from build123d import *

# Parameters (mm, degrees)
SKETCH1_W           = 5
SKETCH1_H           = 38.6
BOSS_EXTRUDE1_DEPTH = 3
SKETCH3_W           = 5
SKETCH3_H           = 15
BOSS_EXTRUDE2_DEPTH = 3
SKETCH4_R           = 1.5
CUT_EXTRUDE1_DEPTH  = 4
SKETCH7_W           = 5
SKETCH7_H           = 15
BOSS_EXTRUDE3_DEPTH = 3
SKETCH8_W           = 5
SKETCH8_H           = 2
BOSS_EXTRUDE4_DEPTH = 12
SKETCH10_W          = 5
SKETCH10_H          = 5
BOSS_EXTRUDE5_DEPTH = 3.65


with BuildPart() as part:
    # Sketch1 → Boss-Extrude1 (new body)
    with BuildSketch(Plane.XY):
        Rectangle(SKETCH1_W, SKETCH1_H)
    extrude(amount=BOSS_EXTRUDE1_DEPTH)

    # Sketch3 → Boss-Extrude2 (add)
    with BuildSketch(Plane.XZ.offset(19.3)):
        with Locations((0, 7.5)):
            Rectangle(SKETCH3_W, SKETCH3_H)
    extrude(amount=BOSS_EXTRUDE2_DEPTH)

    # Sketch4 → Cut-Extrude1 (cut)
    with BuildSketch(Plane(origin=(0, -19.3, 0), x_dir=(1, 0, 0), z_dir=(0, 1, 0))):
        with Locations(Location((0, -9.153210304, 0), (0, 0, 270))):
            Circle(SKETCH4_R)
    extrude(amount=-CUT_EXTRUDE1_DEPTH, mode=Mode.SUBTRACT)

    # Sketch7 → Boss-Extrude3 (add)
    with BuildSketch(Plane(origin=(0, 19.3, 0), x_dir=(1, 0, 0), z_dir=(0, 1, 0))):
        with Locations((0, 4.5)):
            Rectangle(SKETCH7_W, SKETCH7_H)
    extrude(amount=BOSS_EXTRUDE3_DEPTH)

    # Sketch8 → Boss-Extrude4 (add)
    with BuildSketch(Plane(origin=(0, 0, 0), x_dir=(-1, 0, 0), z_dir=(0, 0, -1))):
        with Locations((0, 8.6)):
            Rectangle(SKETCH8_W, SKETCH8_H)
    extrude(amount=BOSS_EXTRUDE4_DEPTH)

    # Sketch10 → Boss-Extrude5 (add)
    with BuildSketch(Plane(origin=(0, 0, 0), x_dir=(-1, 0, 0), z_dir=(0, 0, -1))):
        with Locations((0, -4.864250557)):
            Rectangle(SKETCH10_W, SKETCH10_H)
        with Locations((0, -19.864250557)):
            Rectangle(SKETCH10_W, SKETCH10_H)
    extrude(amount=BOSS_EXTRUDE5_DEPTH)


solid = part.part
Geometry check sheet. Reference: the model listing, model coordinates, mm. A direction names the side the tool comes from. Coordinates: 2 decimals unless noted, no trailing zeros. Order: outer loops, then holes, each group sorted by start corner. A loop starts at its lowest first (then second) coordinate and runs counter-clockwise, first axis right, second up. Notation, with made-up numbers: (-6.75, -22) - (43.25, -22) arc R13 cw to (43.25, 1) - close; hole circle Ø6 at (-29, 3). An arc over 180 degrees is marked (long way). One line per item, written item: value.
(1) Depth check by flat-ended pin: pin 1 Ø2.5 at (x, z) = (0, 9.15) entering from +Y; pin 2 Ø1.5 at (x, y) = (-1, -8) entering from +Z; pin 3 Ø6 at (y, z) = (-4, -4) entering from -X; pin 4 Ø1.5 at (x, y) = (-1, -6) entering from -Z. Enter the tip coordinate at first touch or a pass-through.
Data:
pin 1: passes through
pin 2: stops at z = 3
pin 3: stops at x = -2.5
pin 4: stops at z = -3.65
(2) Sectioned sample at C-C (y = 9). Enter the section's corners in (x, z), and give its area (3 significant figures).
Data:
outline: (-2.5, -12) - (2.5, -12) - (2.5, 3) - (-2.5, 3) - close
area: 75.0 mm^2
(3) Sectioned sample at A-A (x = 0). Enter the section's corners in (y, z), and give its area (3 significant figures).
Data:
outline: (-22.36, -3.65) - (-17.36, -3.65) - (-17.36, 0) - (-7.36, 0) - (-7.36, -3.65) - (-2.36, -3.65) - (-2.36, 0) - (7.6, 0) - (7.6, -12) - (9.6, -12) - (9.6, 0) - (19.3, 0) - (19.3, -12) - (22.3, -12) - (22.3, 3) - (-19.3, 3) - (-19.3, 7.65) - (-22.3, 7.65) - (-22.3, 0) - (-22.36, 0) - close; (-22.3, 10.65) - (-19.3, 10.65) - (-19.3, 15) - (-22.3, 15) - close
area: 257 mm^2
(4) Access from +Z, -Z, +X, -X, +Y, -Y to the whole of each face (thin tool, end or side, straight path). Record for faces 5 (the face through (0, -2.364, -2)), 6 (the face through (0, -5, -3.65)), 7 (the face through (-0.6, -22.3, 7.6)), 8 (the face through (-2, -19.3, 9)).
Data:
face 5: -Z, +X, -X
face 6: -Z, +X, -X, -Y
face 7: +Z, +X, -X, -Y
face 8: +Z, +X, -X, +Y
(5) Sectioned sample at B-B (y = -3). Enter the section's corners in (x, z).
Data:
outline: (-2.5, -3.65) - (2.5, -3.65) - (2.5, 3) - (-2.5, 3) - close
(6) Release check for a two-part mould opening along Z. For faces 1 (the face through (-0.57, -20.78, 10.54)), 2 (the face through (0, 1, 3)), 3 (the face through (0, 3, 0)), 4 (the face through (0, -17.364, -2)) record: +Z half, -Z half, draft (parallel to the pull), parting line (faces both ways), or undercut.
Data:
face 1: undercut
face 2: +Z half
face 3: -Z half
face 4: draft
(7) Thickness scan on probe 1 along Y at (x, z) = (-1, -3.5); probe 2 along Y at (x, z) = (-0.55, -9.5); probe 3 along Z at (x, y) = (0.6, -13). Record the ranges inside material, lowest first. Write a range as from..to.
Data:
probe 1: y = -22.36..-17.36, -7.36..-2.36, 7.6..9.6, 19.3..22.3
probe 2: y = 7.6..9.6, 19.3..22.3
probe 3: z = 0..3
